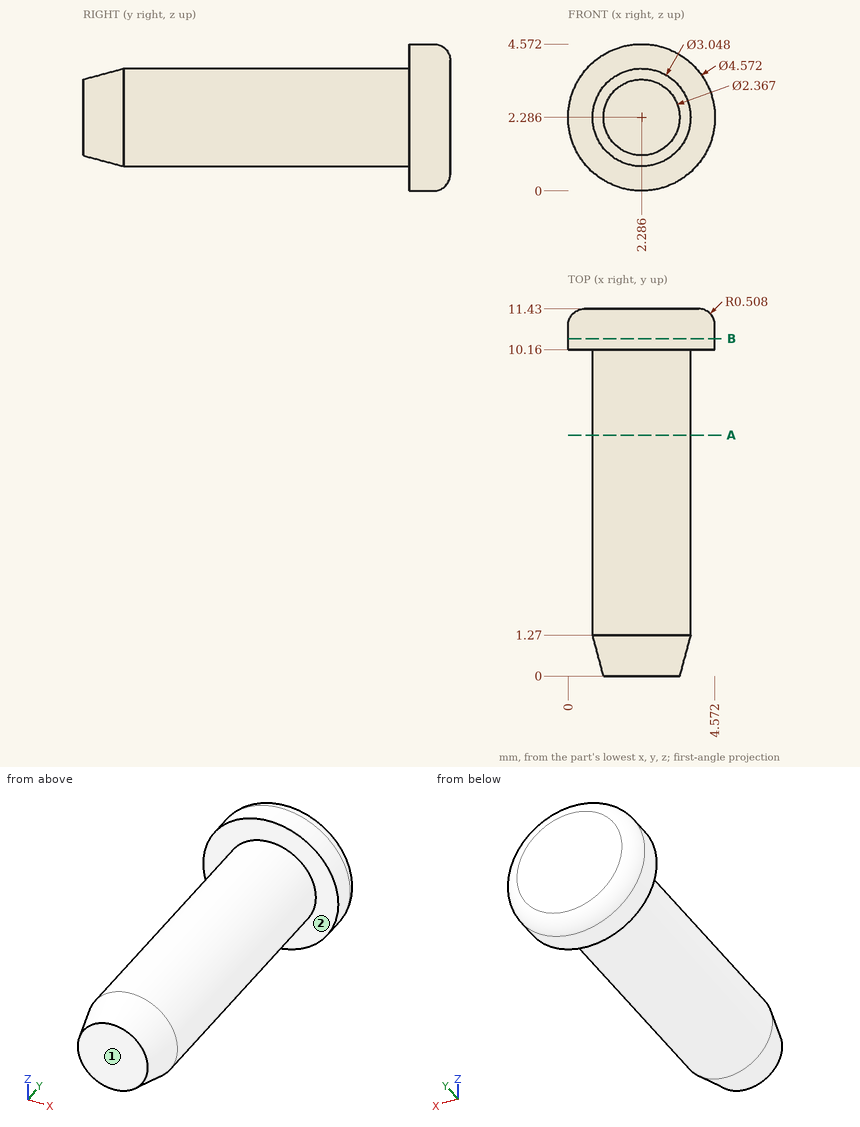
Input: dimensioned drawing with shaded views. Units: mm. Origin: part minimum x, y, z. A direction names the side the tool comes from. Round coordinates to 2 decimals unless told otherwise and drop trailing zeros. Order: outer loops, then holes, each group sorted by start corner. A loop starts at its lowest first (then second) coordinate and runs counter-clockwise, first axis right, second up.
1. Cut plane A-A, the plane y = 7.5. Output: boundary loops of the cut face in (x, z).
The answers:
outline: circle Ø3.05 at (2.29, 2.29)
2. Set-up query: the marked faces 1 and 2. Return all of +Z, -Z, +X, -X, +Y, -Y with unobstructed straight access to the full face (end or side cutting, diameter ignored); none if empty.
The answers:
face 1: +Z, -Z, +X, -X, -Y
face 2: -Y
3. Material intervals for line 1 (Z direction, x = 3.25, y = 3.75) (1 decimal); line 2 (Y direction, x = 3.85, z = 3.1); line 3 (X direction, y = 4.25, z = 1.05) (1 decimal), sorted ascending.
The answers:
line 1: z = 1.1 to 3.5
line 2: y = 10.16 to 11.43
line 3: x = 1.4 to 3.2
4. Cut plane B-B, the plane y = 10.5. Output: boundary loops of the cut face in (x, z), then the cut area to 3 significant figures.
The answers:
outline: circle Ø4.57 at (2.29, 2.29)
area: 16.4 mm2
